Model file for the job. Use its own axes, mm. Round coordinates to 2 decimals unless told otherwise and drop trailing zeros. Write each loop counter-clockwise with the first axis right and the second up, starting at its lowest first coordinate (ties: lowest second). Pieces come first, ordered by that corner, then holes. Notation, with made-up numbers: (-15, 81.25) - (-11, 81.25) arc R24 cw to (-11, 103.25) - close; hole circle Ø7 at (66.5, -10.5). An arc over 180 degrees is marked (long way). One line per item, written item: value.
from build123d import *

# Parameters (mm, degrees)
F0_W     = 60
F0_H     = 40
F1_DEPTH = 15
F2_SIZE  = 1
F3_R     = 5
F3_R_2   = 6
F4_DEPTH = 15.001


with BuildPart() as f1:
    # F0 (on Top) → F1 (new body)
    with BuildSketch(Plane.XY):
        Rectangle(F0_W, F0_H)
    extrude(amount=-F1_DEPTH)

    # F2
    f2_edges = [f1.edges().sort_by_distance(p)[0] for p in [
        (30, 0, 0),
        (0, 20, 0),
        (-30, 0, 0),
        (0, -20, 0),
        (30, 0, -15),
        (0, 20, -15),
        (-30, 0, -15),
        (0, -20, -15),
    ]]
    chamfer(f2_edges, length=F2_SIZE)

    # F3 (on face) → F4 (cut, through all)
    with BuildSketch(Plane.XY):
        with Locations((-20, 0)):
            Circle(F3_R)
        Circle(F3_R_2)
    extrude(amount=-F4_DEPTH, mode=Mode.SUBTRACT)


solid = f1.part
1. Wall check: probe 1 along Y at (x, z) = (0, -5.75); probe 2 along Y at (x, z) = (-20, -5.25). Give the ranges that are in metal, low to high. Write a range as [from, to].
Report:
probe 1: [-20, -6], [6, 20]
probe 2: [-20, -5], [5, 20]
2. Band-saw the part on B-B on y = 0. Write the cut outline in (x, z).
Report:
outline: (-30, -14) - (-29, -15) - (-25, -15) - (-25, 0) - (-29, 0) - (-30, -1) - close; (-15, -15) - (-6, -15) - (-6, 0) - (-15, 0) - close; (6, -15) - (29, -15) - (30, -14) - (30, -1) - (29, 0) - (6, 0) - close
3. Mould opens along X. For faces 1 (the face through (30, 0, -7)), 2 (the face through (-6, 0, -7)), 3 (the face through (0, 20, -7)) say: released by +X, released by -X, zero draft, split by the parting line, or undercut.
Report:
face 1: released by +X
face 2: undercut
face 3: zero draft
4. Band-saw the part on D-D on x = 0. Write the cut outline in (y, z), plus the area to 3 significant figures.
Report:
outline: (-20, -14) - (-19, -15) - (-6, -15) - (-6, 0) - (-19, 0) - (-20, -1) - close; (6, -15) - (19, -15) - (20, -14) - (20, -1) - (19, 0) - (6, 0) - close
area: 418 mm²
5. Band-saw the part on C-C on z = -6. Write the cut outline in (x, y), plus the area to 3 significant figures.
Report:
outline: (-30, -20) - (30, -20) - (30, 20) - (-30, 20) - close; hole circle Ø10 at (-20, 0); hole circle Ø12 at (0, 0)
area: 2,210 mm²
6. Band-saw the part on A-A on x = -20. Write the cut outline in (y, z).
Report:
outline: (-20, -14) - (-19, -15) - (-5, -15) - (-5, 0) - (-19, 0) - (-20, -1) - close; (5, -15) - (19, -15) - (20, -14) - (20, -1) - (19, 0) - (5, 0) - close
